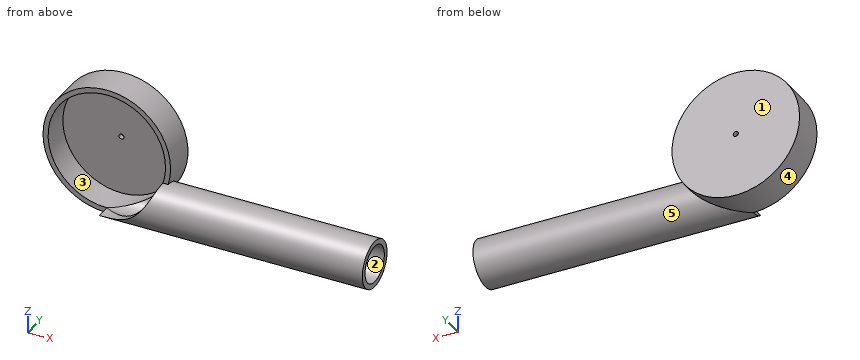
from build123d import *

# Parameters (mm, degrees)
F0_R      = 25
F0_R_2    = 1
F1_DEPTH  = 13
F2_R      = 23
F3_DEPTH  = 11
F4_R      = 9.2
F4_R_2    = 7.2
F5_DEPTH  = 105
F6_DEPTH  = 50.8
F7_DEPTH  = 25.4
F8_R      = 23
F9_DEPTH  = 25.4
F11_ANGLE = 180


with BuildPart() as f1:
    # F0 (on Front) → F1 (new body)
    with BuildSketch(Plane.XZ):
        Circle(F0_R)
        Circle(F0_R_2, mode=Mode.SUBTRACT)
    extrude(amount=F1_DEPTH)

    # F2 (on face) → F3 (cut)
    with BuildSketch(Plane(origin=(0, 0, 0), x_dir=(-1, 0, 0), z_dir=(0, 1, 0))):
        Circle(F2_R)
    extrude(amount=-F3_DEPTH, mode=Mode.SUBTRACT)

    # F4 (on Right) → F5 (join)
    with BuildSketch(Plane.YZ):
        with Locations((0, -15.8)):
            Circle(F4_R)
        with Locations((0, -15.8)):
            Circle(F4_R_2, mode=Mode.SUBTRACT)
    extrude(amount=-F5_DEPTH)

    # F4 (on Right) → F6 (cut)
    with BuildSketch(Plane.YZ):
        with Locations((0, -15.8)):
            Circle(F4_R_2)
    extrude(amount=-F6_DEPTH, mode=Mode.SUBTRACT)

    # F0 (on Front) → F7 (cut)
    with BuildSketch(Plane.XZ):
        Circle(F0_R_2)
    extrude(amount=-F7_DEPTH, mode=Mode.SUBTRACT)

    # F8 (on face) → F9 (cut)
    with BuildSketch(Plane(origin=(0, -11, 0), x_dir=(-1, 0, 0), z_dir=(0, 1, 0))):
        Circle(F8_R)
    extrude(amount=F9_DEPTH, mode=Mode.SUBTRACT)


with BuildPart() as f1_1:
    # F11: moved
    add(f1.part.rotate(Axis((0, 0, 3.9728134871), (0, 0, -1)), F11_ANGLE))


solid = f1_1.part
Part model, mm, in its own coordinate system. Face numbers are marked on the shaded views. A direction names the side the tool comes from. Coordinates: 2 decimals unless noted, no trailing zeros. Loops run counter-clockwise (first coordinate to the right, second up) from the corner with the lowest first, then second, coordinate; pieces in that order, holes last. Notation, with made-up numbers: M 73.25,72.25 L 97.25,72.25 A19 ccw 97.25,82.25 Z; hole C -23.5,50 d3. An arc over 180 degrees is marked long. Use a Markdown table: item, result. Add a question column.
Q1. Cut at A-A (z = -15.8). Write the cut outline in (x, y), and give its area (3 significant figures).
Q2. Probe L1, parallel to X at y = 6.25, z = -1; L2, parallel to Z at x = 0, y = 12.5; L3, parallel to Z at x = 42, y = -0.25. List the from-to ranges inside material, lowest first.
Q3. Cut at D-D (z = 12). Write the cut outline in (x, y).
Q4. Cut at C-C (x = 45). Write the cut outline in (y, z).
Q5. Pin check, flat tips, straight feed: P1, Ø1.8, axis at x = 0, z = 0, coming from the +Y side; P2, Ø8, axis at x = -0.5, z = -4, coming from the -Y side; P3, Ø8, axis at x = 80, y = -1, coming from the +Z side; P4, Ø2, axis at y = -3, z = -24, coming from the -X side. Stop position of each tip, or through.
Q6. Mould opens along Z. For the marked faces 1 and 2 say: +Z half, -Z half, draft (parallel to the pull), parting line (faces both ways), or undercut.
Q7. Which spindle directions (+Z, -Z, +X, -X, +Y, -Y) get a long thin tool onto all of the face, cutting with end or side? Do the marked faces 3, 4 and 5. Say none if no direction does.
Q8. Cut at B-B (y = -2). Write the cut outline in (x, z), and give its area (3 significant figures).
Worked out:
| question | item | result |
|---|---|---|
| 1 | outline | M -19.37,0 L -16.71,0 L -16.71,11 L 16.71,11 L 16.71,7.2 L 105,7.2 L 105,9.2 L 19.37,9.2 L 19.37,13 L -19.37,13 Z; M 16.71,-9.2 L 105,-9.2 L 105,-7.2 L 16.71,-7.2 Z |
| 1 | area | 465 mm2 |
| 2 | L1 | x = -24.98 to -22.98, 22.98 to 24.98 |
| 2 | L2 | z = -25 to -1, 1 to 25 |
| 2 | L3 | z = -25 to -23, -8.6 to -6.6 |
| 3 | outline | M -21.93,0 L -19.62,0 L -19.62,11 L 19.62,11 L 19.62,0 L 21.93,0 L 21.93,13 L -21.93,13 Z |
| 4 | outline | C 0,-15.8 d18.4; hole C 0,-15.8 d14.4 |
| 5 | P1 | passes through |
| 5 | P2 | stops at y = 11 |
| 5 | P3 | stops at z = -6.6 |
| 5 | P4 | stops at x = 0 |
| 6 | face 1 | draft |
| 6 | face 2 | undercut |
| 7 | face 3 | -Y |
| 7 | face 4 | +Y |
| 7 | face 5 | +X |
| 8 | outline | M 0,-24.78 L 105,-24.78 L 105,-22.72 L 3.6,-22.72 A23 cw 0,-23 Z; M 21.22,-8.88 L 105,-8.88 L 105,-6.82 L 21.97,-6.82 A23 cw Z |
| 8 | area | 388 mm2 |
